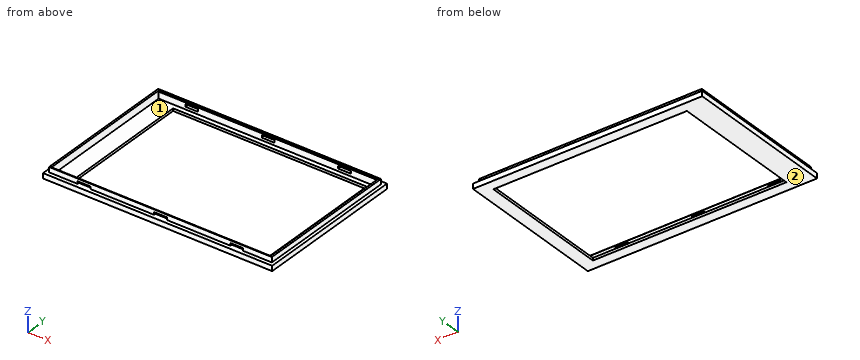
```python
from build123d import *

# Parameters (mm, degrees)
SKETCH_W      = 90
SKETCH_H      = 60
SKETCH_W_2    = 76
SKETCH_H_2    = 52
PAD_DEPTH     = 1
SKETCH001_W   = 90
SKETCH001_H   = 60
SKETCH001_W_2 = 86
SKETCH001_H_2 = 55.6
PAD001_DEPTH  = 1
SKETCH002_W   = 87.5
SKETCH002_H   = 57
SKETCH002_W_2 = 86
SKETCH002_H_2 = 55.6
PAD002_DEPTH  = 2
SKETCH003_W   = 5
SKETCH003_H   = 1
POCKET_DEPTH  = 58.501
CHAMFER_SIZE  = 0.4


with BuildPart() as part:
    # Sketch → Pad (new body)
    with BuildSketch(Plane.XY):
        Rectangle(SKETCH_W, SKETCH_H)
        with Locations((2, 0)):
            Rectangle(SKETCH_W_2, SKETCH_H_2, mode=Mode.SUBTRACT)
    extrude(amount=PAD_DEPTH)

    # Sketch001 → Pad001 (new body)
    with BuildSketch(Plane.XY.offset(1)):
        Rectangle(SKETCH001_W, SKETCH001_H)
        Rectangle(SKETCH001_W_2, SKETCH001_H_2, mode=Mode.SUBTRACT)
    extrude(amount=PAD001_DEPTH)

    # Sketch002 → Pad002 (new body)
    with BuildSketch(Plane.XY.offset(2)):
        Rectangle(SKETCH002_W, SKETCH002_H)
        Rectangle(SKETCH002_W_2, SKETCH002_H_2, mode=Mode.SUBTRACT)
    extrude(amount=PAD002_DEPTH)

    # Sketch003 → Pocket (cut, through all)
    with BuildSketch(Plane.XZ.offset(28.5)):
        with Locations((-30, 2.5)):
            Rectangle(SKETCH003_W, SKETCH003_H)
        with Locations((0, 2.5)):
            Rectangle(SKETCH003_W, SKETCH003_H)
        with Locations((30, 2.5)):
            Rectangle(SKETCH003_W, SKETCH003_H)
    extrude(amount=-POCKET_DEPTH, mode=Mode.SUBTRACT)

    # Chamfer
    chamfer_edges = [part.edges().sort_by_distance(p)[0] for p in [
        (0, 27.8, 4),
        (0, -27.8, 4),
    ]]
    chamfer(chamfer_edges, length=CHAMFER_SIZE)


solid = part.part
```
Work out the finished part from the listing and answer in its coordinate system (mm). Face numbers are marked on the shaded views. Round coordinates to 2 decimals unless told otherwise and drop trailing zeros. Loops run counter-clockwise (first coordinate to the right, second up) from the corner with the lowest first, then second, coordinate; pieces in that order, holes last. Notation, with made-up numbers: (86.5, 83.5) -> (137.5, 83.5) arc R18 ccw to (137.5, 116.5) -> close; hole circle Ø6 at (79.5, 71). An arc over 180 degrees is marked (long way). Write each question's results on one line, items separated by ' | '. Start each with the question number.
1. Section A-A (x = 17.5) is taken. Determine the outline of the cut face in (y, z), plus the area to 3 significant figures.
2. Section B-B (y = -8.5) is taken. Determine the outline of the cut face in (x, z).
3. For a pull along Y with two mould halves and no side action, classify the marked faces 1 and 2 as +Y half, -Y half, draft (parallel to the pull), parting line (faces both ways), or undercut.
4. Given pin 1 Ø1.6 at (y, z) = (1.5, 3) entering from -X; pin 2 Ø0.8 at (y, z) = (28, 2.5) entering from +X; pin 3 Ø1 at (x, z) = (-4, 3) entering from +Y, each flat-ended and moving along its own axis, determine where each tip first touches the part or whether it passes through.
5. Find the intervals of material crossed by probe 1 along X at (y, z) = (19, 2.2); probe 2 along Y at (x, z) = (19.5, 0.8); probe 3 along X at (y, z) = (-18, 1.15), in increasing order. Write a range as from..to.
Evaluation:
1) outline: (-30, 0) -> (-26, 0) -> (-26, 1) -> (-27.8, 1) -> (-27.8, 3.6) -> (-28.2, 4) -> (-28.5, 4) -> (-28.5, 2) -> (-30, 2) -> close; (26, 0) -> (30, 0) -> (30, 2) -> (28.5, 2) -> (28.5, 4) -> (28.2, 4) -> (27.8, 3.6) -> (27.8, 1) -> (26, 1) -> close | area: 15.0 mm2
2) outline: (-45, 0) -> (-36, 0) -> (-36, 1) -> (-43, 1) -> (-43, 4) -> (-43.75, 4) -> (-43.75, 2) -> (-45, 2) -> close; (40, 0) -> (45, 0) -> (45, 2) -> (43.75, 2) -> (43.75, 4) -> (43, 4) -> (43, 1) -> (40, 1) -> close
3) face 1: undercut | face 2: draft
4) pin 1: stops at x = -43.75 | pin 2: stops at x = 43.75 | pin 3: stops at y = 28.5
5) probe 1: x = -43.75..-43, 43..43.75 | probe 2: y = -30..-26, 26..30 | probe 3: x = -45..-43, 43..45
